Design review of the part shown in the three views and the two pictorial views. Dimensions are in mm from the part's minimum x, y and z. Round coordinates to 2 decimals unless told otherwise and drop trailing zeros. Order: outer loops, then holes, each group sorted by start corner. A loop starts at its lowest first (then second) coordinate and runs counter-clockwise, first axis right, second up. Notation, with made-up numbers: M -17.75,70.5 L 15.25,70.5 A9 ccw 15.25,80.5 Z; hole C 67.5,6 d4. An arc over 180 degrees is marked long. Use a Markdown table: item, result. Add a question column.
(1) For pin 1 (10 mm diameter, centred on x = 20.5, z = 107, fed in from -Y); pin 2 (1.5 mm diameter, centred on y = 2, z = 51, fed in from +X); pin 3 (0.9 mm diameter, centred on y = 1, z = 84, fed in from -X); pin 4 (1.5 mm diameter, centred on x = 55, y = 1.5, fed in from +Z), all flat-tipped, find the tip position at first contact; note any pin that passes through.
(2) Take a section at A-A (y = 1.5). Write out the cut boundary in (x, z), then the cut area to 3 significant figures.
(3) To check wall thickness, follow probe 1 along Z at (x, y) = (63.5, 1.3); probe 2 along X at (y, z) = (1.5, 31); probe 3 along Z at (x, y) = (85.5, 2.15). State the ranges of each line that lie inside material, in increasing order. Write a range as from..to.
(4) Take a section at B-B (x = 47). Write out the cut boundary in (y, z), then the cut area to 3 significant figures.
(5) Take a section at C-C (z = 76). Write out the cut boundary in (x, y), then the cut area to 3 significant figures.
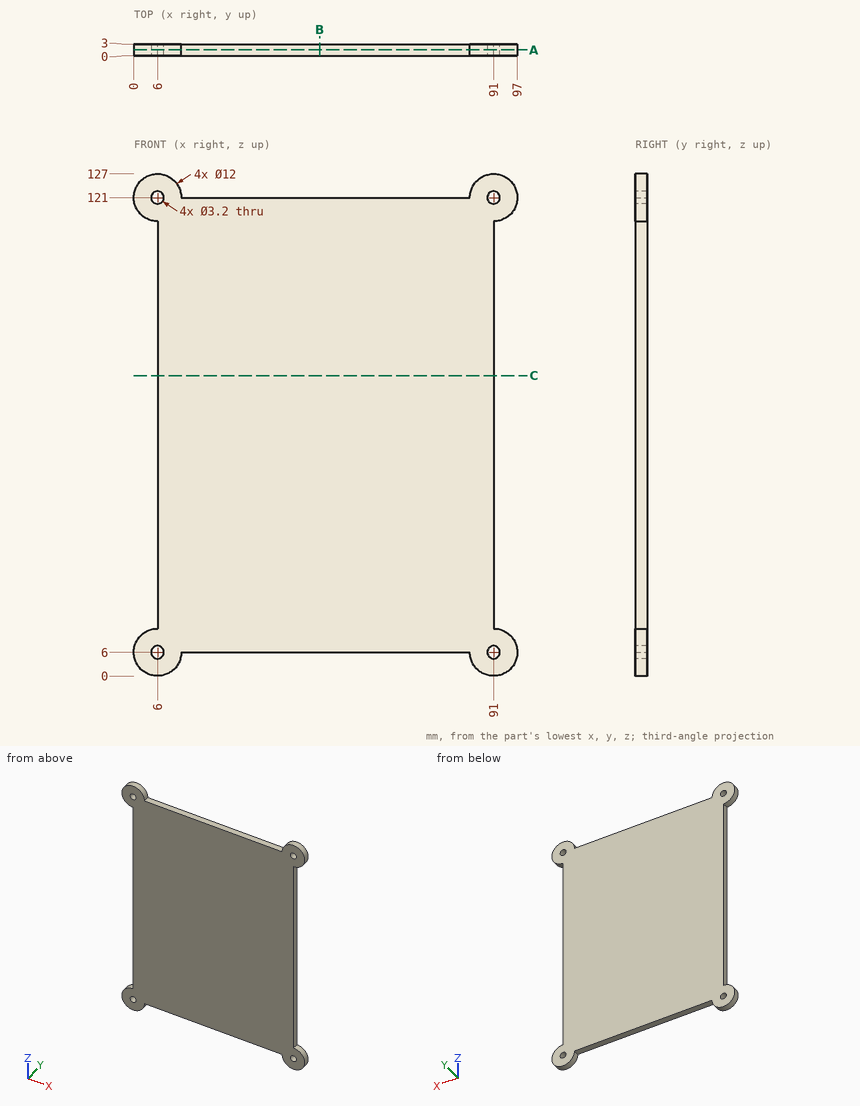
Verdict:
| question | item | result |
|---|---|---|
| 1 | pin 1 | stops at y = 0 |
| 1 | pin 2 | stops at x = 91 |
| 1 | pin 3 | stops at x = 6 |
| 1 | pin 4 | stops at z = 121 |
| 2 | outline | M 6,12 A6 ccw long 12,6 L 85,6 A6 ccw long 91,12 L 91,115 A6 ccw long 85,121 L 12,121 A6 ccw long 6,115 Z; hole C 6,6 d3.2; hole C 6,121 d3.2; hole C 91,6 d3.2; hole C 91,121 d3.2 |
| 2 | area | 10,100 mm^2 |
| 3 | probe 1 | z = 6..121 |
| 3 | probe 2 | x = 6..91 |
| 3 | probe 3 | z = 3.6..123.4 |
| 4 | outline | M 0,6 L 3,6 L 3,121 L 0,121 Z |
| 4 | area | 345 mm^2 |
| 5 | outline | M 6,0 L 91,0 L 91,3 L 6,3 Z |
| 5 | area | 255 mm^2 |
